The model under review builds one solid part; all positions refer to its coordinate system, in mm. A direction names the side the tool comes from. Coordinates: 2 decimals unless noted, no trailing zeros. Order: outer loops, then holes, each group sorted by start corner. A loop starts at its lowest first (then second) coordinate and runs counter-clockwise, first axis right, second up.
```python
from build123d import *

# Parameters (mm, degrees)
SWEEP1_PROFILE_R     = 6.35
CUT_SWEEP1_PROFILE_R = 3.175


with BuildPart() as part:
    # Sweep1: sweep along a curve in space
    with BuildLine() as sweep1_path:
        Line((0, 50.8, 340.36), (0, 76.2, 340.36))
        ThreePointArc((0, 12.7, 302.26), (0, 23.859231637, 329.200768363), (0, 50.8, 340.36))
        Line((0, 12.7, 302.26), (0, 12.7, -2.54))
    # Sweep1 profile (on start of the path) → Sweep1 (sweep)
    with BuildSketch(Plane(origin=(0, 12.7, -2.54), x_dir=(1, 0, 0), z_dir=(0, 0, 1))):
        Circle(SWEEP1_PROFILE_R)
    sweep(path=sweep1_path.line)

    # Cut-Sweep1: sweep along a curve in space
    with BuildLine() as cut_sweep1_path:
        Line((0, 50.8, 340.36), (0, 76.2, 340.36))
        ThreePointArc((0, 12.7, 302.26), (0, 23.859231637, 329.200768363), (0, 50.8, 340.36))
        Line((0, 12.7, 302.26), (0, 12.7, -2.54))
    # Cut-Sweep1 profile (on start of the path) → Cut-Sweep1 (sweep, cut)
    with BuildSketch(Plane(origin=(0, 12.7, -2.54), x_dir=(1, 0, 0), z_dir=(0, 0, 1))):
        Circle(CUT_SWEEP1_PROFILE_R)
    sweep(path=cut_sweep1_path.line, mode=Mode.SUBTRACT)


solid = part.part
```
(1) For pin 1 Ø1 at (x, y) = (2.5, 63.5) entering from +Z; pin 2 Ø5 at (x, z) = (3, 43) entering from -Y; pin 3 Ø6 at (x, y) = (2.5, 34.5) entering from -Z, all flat-tipped, find the tip position at first contact; note any pin that passes through.
A:
pin 1: stops at z = 346.39
pin 2: stops at y = 6.37
pin 3: stops at z = 327.82
(2) Wall thickness on probe 1 along Y at (x, z) = (0, 140) (3 decimals); probe 2 along Z at (x, y) = (0.5, 50); probe 3 along Z at (x, y) = (-1.25, 24.5): over which ranges is each line inside the solid? List them lowest first.
A:
probe 1: y = 6.35 to 9.525, 15.875 to 19.05
probe 2: z = 334.02 to 337.22, 343.49 to 346.68
probe 3: z = 320.27 to 325.63, 333.74 to 337.94
(3) We need section C-C, the plane y = 54.5. Write out the cut boundary in (x, z) (3 decimals), and give its area (3 significant figures).
A:
outline: circle Ø12.7 at (0, 340.36); hole circle Ø6.35 at (0, 340.36)
area: 95.0 mm2
(4) We need section B-B, the plane z = 23.5. Write out the cut boundary in (x, y) (3 decimals).
A:
outline: circle Ø12.7 at (0, 12.7); hole circle Ø6.35 at (0, 12.7)
(5) Draft analysis for pull direction Y (two halves, no side actions). For faces 3 (the face through (1.5, 9.9, 152)), 4 (the face through (-0.69, 63.68, 343.46)), 5 (the face through (3.414, 18.054, 151.994)), state which applies: released by +Y, released by -Y, zero draft, split by the parting line, or undercut.
A:
face 3: undercut
face 4: zero draft
face 5: split by the parting line
(6) We need section A-A, the plane x = 0. Write out the cut boundary in (y, z) (3 decimals), and give its area (3 significant figures).
A:
outline: (6.35, -2.54) - (9.525, -2.54) - (9.525, 302.26) arc R41.275 cw to (50.8, 343.535) - (76.2, 343.535) - (76.2, 346.71) - (50.8, 346.71) arc R44.45 ccw to (6.35, 302.26) - close; (15.875, -2.54) - (19.05, -2.54) - (19.05, 302.26) arc R31.75 cw to (50.8, 334.01) - (76.2, 334.01) - (76.2, 337.185) - (50.8, 337.185) arc R34.925 ccw to (15.875, 302.26) - close
area: 2,480 mm2
(7) Machinability: for faces 1 (the face through (3, 76.2, 342)), 2 (the face through (-1.38, 63.68, 346.56)), which of the approach directions +Z, -Z, +X, -X, +Y, -Y give a long, thin tool a straight path to every point of the face, cutting with its end or side? Answer none if there is none.
A:
face 1: +Z, -Z, +X, -X, +Y
face 2: +Y
